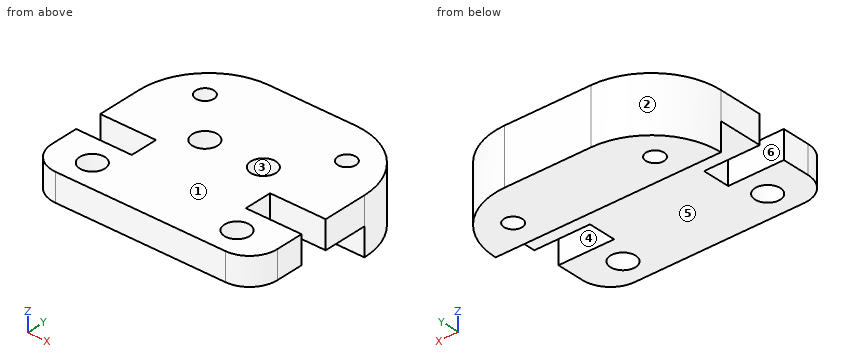
from build123d import *

# Parameters (mm, degrees)
SKETCH1_R           = 0.9
SKETCH1_R_2         = 0.65
BOSS_EXTRUDE1_DEPTH = 4
SKETCH2_W           = 16.2
SKETCH2_H           = 9.205
CUT_EXTRUDE1_DEPTH  = 2


with BuildPart() as part:
    # Sketch1 → Boss-Extrude1 (new body)
    with BuildSketch(Plane.XY):
        with BuildLine():
            Line((12.2, 4), (16.2, 4))
            Line((16.2, 4), (16.2, 2))
            ThreePointArc((16.2, 2), (15.614213562, 0.585786438), (14.2, 0))
            Line((14.2, 0), (2, 0))
            ThreePointArc((2, 0), (0.585786438, 0.585786438), (0, 2))
            Line((0, 2), (0, 4))
            Line((0, 4), (4, 4))
            Line((4, 4), (4, 6))
            Line((4, 6), (0, 6))
            Line((0, 6), (0, 9.205))
            ThreePointArc((0, 9.205), (1.464466094, 12.740533906), (5, 14.205))
            Line((5, 14.205), (11.2, 14.205))
            ThreePointArc((11.2, 14.205), (14.735533906, 12.740533906), (16.2, 9.205))
            Line((16.2, 9.205), (16.2, 6))
            Line((16.2, 6), (12.2, 6))
            Line((12.2, 6), (12.2, 4))
        make_face()
        with Locations((13.3, 2)):
            Circle(SKETCH1_R, mode=Mode.SUBTRACT)
        with Locations((13.2, 11.205)):
            Circle(SKETCH1_R_2, mode=Mode.SUBTRACT)
        with Locations((10.2, 7.75)):
            Circle(SKETCH1_R, mode=Mode.SUBTRACT)
        with Locations((6, 7.75)):
            Circle(SKETCH1_R, mode=Mode.SUBTRACT)
        with Locations((3, 11.205)):
            Circle(SKETCH1_R_2, mode=Mode.SUBTRACT)
        with Locations((2.9, 2)):
            Circle(SKETCH1_R, mode=Mode.SUBTRACT)
    extrude(amount=BOSS_EXTRUDE1_DEPTH)

    # Sketch2 → Cut-Extrude1 (cut)
    with BuildSketch(Plane(origin=(0, 0, 0), x_dir=(-1, 0, 0), z_dir=(0, 0, -1))):
        with Locations((-8.1, 4.6025)):
            Rectangle(SKETCH2_W, SKETCH2_H)
    extrude(amount=-CUT_EXTRUDE1_DEPTH, mode=Mode.SUBTRACT)


solid = part.part
Geometry: final body of the model. Coordinates: model frame, mm. Face numbers are marked on the shaded views. A direction names the side the tool comes from. Round coordinates to 2 decimals unless told otherwise and drop trailing zeros. Loops run counter-clockwise (first coordinate to the right, second up) from the corner with the lowest first, then second, coordinate; pieces in that order, holes last.
Q1. Section A-A on x = 6. Return loops of the section in (y, z) (3 decimals).
Q2. Access query for the marked faces 4, 5 and 6. Directions: +Z, -Z, +X, -X, +Y, -Y. A direction counts if a zero-diameter tool reaches every point of the face in a straight line with its end or side. Return the directions, or none.
Q3. Pull-direction query (X, two-part tool) for the marked faces 1, 2 and 3; classes: released by +X, released by -X, zero draft, split by the parting line, or undercut.
Q4. Material intervals for L1, parallel to X at y = 2, z = 2.6; L2, parallel to X at y = 7.75, z = 2.75; L3, parallel to Z at x = 8.25, y = 8.5, sorted ascending.
Q5. Section D-D on z = 1.1. Return loops of the section in (x, y) (3 decimals).
Q6. Section C-C on x = 13.3. Return loops of the section in (y, z) (3 decimals), plus the area to 3 significant figures.
Q7. Pin query (flat end, axial travel): P1, Ø2, axis at x = 6, y = 7.75, coming from the -Z side; P2, Ø1.1, axis at x = 13.3, y = 2, coming from the -Z side; P3, Ø2, axis at x = 2, z = 2.5, coming from the +Y side; P4, Ø1.6, axis at x = 15, z = 2.5, coming from the +Y side (3 decimals). Return the tip coordinate at first contact, or that it passes through.
Q8. Section B-B on y = 7.25. Return loops of the section in (x, z).
Evaluation:
1. outline: (0, 2) - (6.85, 2) - (6.85, 4) - (0, 4) - close; (8.65, 2) - (9.205, 2) - (9.205, 0) - (14.205, 0) - (14.205, 4) - (8.65, 4) - close
2. face 4: +Z, -Z, +X
2. face 5: -Z, +X, -X, -Y
2. face 6: +Z, -Z, -X
3. face 1: zero draft
3. face 2: released by -X
3. face 3: undercut
4. L1: x = 0 to 2, 3.8 to 12.4, 14.2 to 16.2
4. L2: x = 0 to 5.1, 6.9 to 9.3, 11.1 to 16.2
4. L3: z = 2 to 4
5. outline: (0, 9.205) - (16.2, 9.205) arc R5 ccw to (11.2, 14.205) - (5, 14.205) arc R5 ccw to start; hole circle Ø1.3 at (3, 11.205); hole circle Ø1.3 at (13.2, 11.205)
6. outline: (0, 2) - (1.1, 2) - (1.1, 4) - (0, 4) - close; (2.9, 2) - (4, 2) - (4, 4) - (2.9, 4) - close; (6, 2) - (9.205, 2) - (9.205, 0) - (10.563, 0) - (10.563, 4) - (6, 4) - close; (11.847, 0) - (13.743, 0) - (13.743, 4) - (11.847, 4) - close
6. area: 23.8 mm2
7. P1: stops at z = 2
7. P2: passes through
7. P3: stops at y = 13.79
7. P4: stops at y = 13.205
8. outline: (0, 2) - (5.25, 2) - (5.25, 4) - (0, 4) - close; (6.75, 2) - (9.45, 2) - (9.45, 4) - (6.75, 4) - close; (10.95, 2) - (16.2, 2) - (16.2, 4) - (10.95, 4) - close
